The listing builds one solid part. Answer for the finished solid, in the listing's coordinates (mm). Face numbers are marked on the shaded views. A direction names the side the tool comes from. Coordinates: 2 decimals unless noted, no trailing zeros. Write each loop counter-clockwise with the first axis right and the second up, starting at its lowest first coordinate (ties: lowest second). Pieces come first, ordered by that corner, then holes.
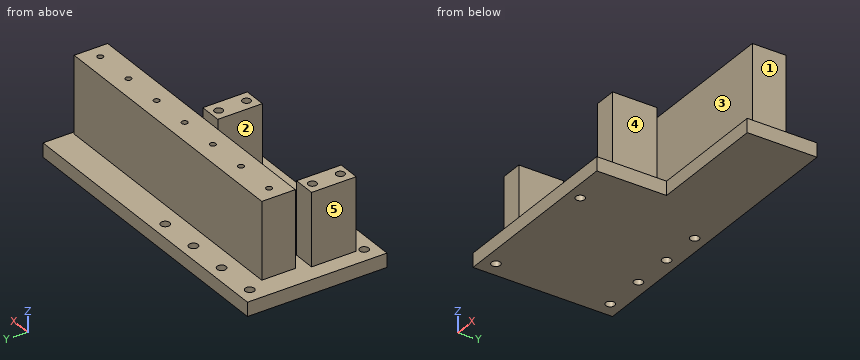
from build123d import *

# Parameters (mm, degrees)
BASE_START                = -5
BASE_PLATE_DEPTH          = 5
MOUNTING_START            = -5.1
MOUNTING_HOLES_PROFILE_R  = 1.6
MOUNTING_HOLES_DEPTH      = 5.3
RAIL_SUPPORT_PROFILE_W    = 100
RAIL_SUPPORT_PROFILE_H    = 12
RAIL_SUPPORT_DEPTH        = 27.5
RAIL_START                = 21
RAIL_FASTENERS_PROFILE_R  = 1.05
RAIL_FASTENERS_DEPTH      = 6.6
SERVO_SUPPORTS_PROFILE_W  = 8
SERVO_SUPPORTS_PROFILE_H  = 16
SERVO_SUPPORTS_DEPTH      = 26
SERVO_START               = 18
SERVO_FASTENERS_PROFILE_R = 1.5
SERVO_FASTENERS_DEPTH     = 8.1


with BuildPart() as part:
    # Base plate profile → Base plate (new body)
    with BuildSketch(Plane.XY.offset(BASE_START)):
        Polygon((-25, -15), (41, -15), (41, 10), (84, 10), (84, 35), (10, 35), (-10, 35), (-25, 35), align=None)
    extrude(amount=BASE_PLATE_DEPTH)

    # Mounting holes profile → Mounting holes (cut)
    with BuildSketch(Plane.XY.offset(MOUNTING_START)):
        with Locations((-19.5, -10.5)):
            Circle(MOUNTING_HOLES_PROFILE_R)
        with Locations((-19.5, 30.5)):
            Circle(MOUNTING_HOLES_PROFILE_R)
        with Locations((25.5, -10.5)):
            Circle(MOUNTING_HOLES_PROFILE_R)
        with Locations((25.5, 30.5)):
            Circle(MOUNTING_HOLES_PROFILE_R)
        with Locations((-4.5, 30.5)):
            Circle(MOUNTING_HOLES_PROFILE_R)
        with Locations((10.5, 30.5)):
            Circle(MOUNTING_HOLES_PROFILE_R)
    extrude(amount=MOUNTING_HOLES_DEPTH, mode=Mode.SUBTRACT)

    # Rail support profile → Rail support (add)
    with BuildSketch(Plane.XY):
        with Locations((33, 18.5)):
            Rectangle(RAIL_SUPPORT_PROFILE_W, RAIL_SUPPORT_PROFILE_H)
    extrude(amount=RAIL_SUPPORT_DEPTH)

    # Rail fasteners profile → Rail fasteners (cut)
    with BuildSketch(Plane.XY.offset(RAIL_START)):
        with Locations((-12, 18.5)):
            Circle(RAIL_FASTENERS_PROFILE_R)
        with Locations((3, 18.5)):
            Circle(RAIL_FASTENERS_PROFILE_R)
        with Locations((18, 18.5)):
            Circle(RAIL_FASTENERS_PROFILE_R)
        with Locations((33, 18.5)):
            Circle(RAIL_FASTENERS_PROFILE_R)
        with Locations((48, 18.5)):
            Circle(RAIL_FASTENERS_PROFILE_R)
        with Locations((63, 18.5)):
            Circle(RAIL_FASTENERS_PROFILE_R)
        with Locations((78, 18.5)):
            Circle(RAIL_FASTENERS_PROFILE_R)
    extrude(amount=RAIL_FASTENERS_DEPTH, mode=Mode.SUBTRACT)

    # Servo supports profile → Servo supports (add)
    with BuildSketch(Plane.XY):
        with Locations((-15, 0)):
            Rectangle(SERVO_SUPPORTS_PROFILE_W, SERVO_SUPPORTS_PROFILE_H)
        with Locations((35, 0)):
            Rectangle(SERVO_SUPPORTS_PROFILE_W, SERVO_SUPPORTS_PROFILE_H)
    extrude(amount=SERVO_SUPPORTS_DEPTH)

    # Servo fasteners profile → Servo fasteners (cut)
    with BuildSketch(Plane.XY.offset(SERVO_START)):
        with Locations((-15, -5)):
            Circle(SERVO_FASTENERS_PROFILE_R)
        with Locations((-15, 5)):
            Circle(SERVO_FASTENERS_PROFILE_R)
        with Locations((35, -5)):
            Circle(SERVO_FASTENERS_PROFILE_R)
        with Locations((35, 5)):
            Circle(SERVO_FASTENERS_PROFILE_R)
    extrude(amount=SERVO_FASTENERS_DEPTH, mode=Mode.SUBTRACT)


solid = part.part
1. Section A-A on z = 2.5 is taken. Give the vertices of the cut face in (x, y), then the cut area to 3 significant figures.
Results found:
outline: (-19, -8) - (-11, -8) - (-11, 8) - (-19, 8) - close; (-17, 12.5) - (83, 12.5) - (83, 24.5) - (-17, 24.5) - close; (31, -8) - (39, -8) - (39, 8) - (31, 8) - close
area: 1,460 mm2
2. A tool of negligible diameter and unlimited length cuts with its end or side. For the marked faces 1, 2, 3, 4 and 5, from which of +Z, -Z, +X, -X, +Y, -Y can it reach the whole face along a straight path? Write none if from no direction.
Results found:
face 1: +Z, +X, +Y, -Y
face 2: +Z, -Y
face 3: +Z, +X, -X
face 4: +Z, +X, -Y
face 5: +Z, -X, +Y, -Y
3. Find the intervals of material crossed by L1, parallel to Y at x = 25.5, z = -1.25; L2, parallel to X at y = -3.5, z = 6.5; L3, parallel to Y at x = 35, z = 23, in increasing order.
Results found:
L1: y = -15 to -12.1, -8.9 to 28.9, 32.1 to 35
L2: x = -19 to -11, 31 to 39
L3: y = -8 to -6.5, -3.5 to 3.5, 6.5 to 8, 12.5 to 24.5
4. Section B-B on x = -4.5 is taken. Give the vertices of the cut face in (y, z), then the cut area to 3 significant figures.
Results found:
outline: (-15, -5) - (28.9, -5) - (28.9, 0) - (24.5, 0) - (24.5, 27.5) - (12.5, 27.5) - (12.5, 0) - (-15, 0) - close; (32.1, -5) - (35, -5) - (35, 0) - (32.1, 0) - close
area: 564 mm2
5. Section D-D on x = 63 is taken. Give the vertices of the cut face in (y, z).
Results found:
outline: (10, -5) - (35, -5) - (35, 0) - (24.5, 0) - (24.5, 27.5) - (19.55, 27.5) - (19.55, 21) - (17.45, 21) - (17.45, 27.5) - (12.5, 27.5) - (12.5, 0) - (10, 0) - close
6. Flat-ended cylindrical pins translate along their axes: P1, Ø3.5, axis at x = -15, y = 5, coming from the +Z side; P2, Ø1, axis at x = 48.5, y = 18.5, coming from the +Z side; P3, Ø6, axis at x = 54.5, y = 29.5, coming from the +Z side. Find the tip coordinate at first contact, or state that the pin passes through.
Results found:
P1: stops at z = 26
P2: stops at z = 21
P3: stops at z = 0
7. Section C-C on y = -5 is taken. Give the vertices of the cut face in (x, z), then the cut area to 3 significant figures.
Results found:
outline: (-25, -5) - (41, -5) - (41, 0) - (39, 0) - (39, 26) - (36.5, 26) - (36.5, 18) - (33.5, 18) - (33.5, 26) - (31, 26) - (31, 0) - (-11, 0) - (-11, 26) - (-13.5, 26) - (-13.5, 18) - (-16.5, 18) - (-16.5, 26) - (-19, 26) - (-19, 0) - (-25, 0) - close
area: 698 mm2
